```python
from build123d import *

# Parameters (mm, degrees)
BOSS_EXTRUDE1_DEPTH = 2
SKETCH3_R           = 10
CUT_EXTRUDE2_DEPTH  = 2
SKETCH2_R           = 1.75
CUT_EXTRUDE1_DEPTH  = 2
SKETCH4_R           = 1.75
CUT_EXTRUDE3_DEPTH  = 2
CIRPATTERN1_COUNT   = 4


with BuildPart() as part:
    # Sketch1 → Boss-Extrude1 (new body)
    with BuildSketch(Plane(origin=(0, 0, 0), x_dir=(1, 0, 0), z_dir=(0, 1, 0))):
        Polygon((-25, 50), (25, 50), (50, 25), (50, -25), (25, -50), (-25, -50), (-50, -25), (-50, 25), align=None)
    extrude(amount=BOSS_EXTRUDE1_DEPTH)

    # Sketch3 → Cut-Extrude2 (cut)
    with BuildSketch(Plane(origin=(0, 2, 0), x_dir=(1, 0, 0), z_dir=(0, 1, 0))):
        Circle(SKETCH3_R)
    extrude(amount=-CUT_EXTRUDE2_DEPTH, mode=Mode.SUBTRACT)

    # Sketch2 → Cut-Extrude1 (cut)
    with BuildSketch(Plane(origin=(0, 2, 0), x_dir=(1, 0, 0), z_dir=(0, 1, 0))):
        with Locations((-45, 20)):
            Circle(SKETCH2_R)
        with Locations((-45, 12)):
            Circle(SKETCH2_R)
        with Locations((-45, 4)):
            Circle(SKETCH2_R)
        with Locations((-45, -4)):
            Circle(SKETCH2_R)
        with Locations((-45, -12)):
            Circle(SKETCH2_R)
        with Locations((-45, -20)):
            Circle(SKETCH2_R)
    cut_extrude1 = extrude(amount=-CUT_EXTRUDE1_DEPTH, mode=Mode.SUBTRACT)

    # Sketch4 → Cut-Extrude3 (cut)
    with BuildSketch(Plane(origin=(0, 2, 0), x_dir=(1, 0, 0), z_dir=(0, 1, 0))):
        with Locations((-29.721825407, 38.207106781)):
            Circle(SKETCH4_R)
        with Locations((-24.064971157, 32.550252532)):
            Circle(SKETCH4_R)
        with Locations((-18.408116908, 26.893398282)):
            Circle(SKETCH4_R)
        with Locations((-12.751262658, 21.236544033)):
            Circle(SKETCH4_R)
        with Locations((-7.094408409, 15.579689783)):
            Circle(SKETCH4_R)
        with Locations((-15.579689783, 7.094408409)):
            Circle(SKETCH4_R)
        with Locations((-21.236544033, 12.751262658)):
            Circle(SKETCH4_R)
        with Locations((-26.893398282, 18.408116908)):
            Circle(SKETCH4_R)
        with Locations((-32.550252532, 24.064971157)):
            Circle(SKETCH4_R)
        with Locations((-38.207106781, 29.721825407)):
            Circle(SKETCH4_R)
        Polygon((-30.959262274, 29.898602102), (-16.81712665, 15.756466479), (-15.756466479, 16.81712665), (-29.898602102, 30.959262274), align=None)
        Polygon((-35, 16), (-20, 1), (-20, -1), (-35, -16), align=None)
    cut_extrude3 = extrude(amount=-CUT_EXTRUDE3_DEPTH, mode=Mode.SUBTRACT)

    # CirPattern1: Cut-Extrude1, Cut-Extrude3 ×4 about axis
    cirpattern1_axis = Axis((0, 0, 0), (0, 1, 0))
    for i in range(1, CIRPATTERN1_COUNT):
        add(cut_extrude1.rotate(cirpattern1_axis, i * 360 / CIRPATTERN1_COUNT), mode=Mode.SUBTRACT)
        add(cut_extrude3.rotate(cirpattern1_axis, i * 360 / CIRPATTERN1_COUNT), mode=Mode.SUBTRACT)


solid = part.part
```
Could you check a few things on this model? Use its own coordinates, in mm. Give positions to 0.01 mm unless a question says otherwise; leave off trailing zeros. Order: outer loops, then holes, each group sorted by start corner. A loop starts at its lowest first (then second) coordinate and runs counter-clockwise, first axis right, second up.
Q1. Suppose I cut it at A-A, the plane z = 45. Write out the boundary of the cut face in (x, y).
Q2. Suppose I cut it at B-B, the plane x = 45. Write out the boundary of the cut face in (y, z), and give its area (3 significant figures).
Q3. If I drill on line 1 along Z through (x, y) = (0, 1.6); line 2 along X through (y, z) = (1.3, 39); line 3 along X through (y, z) = (1.4, -32.5), over which ranges is the centre line in solid material (lowest first)?
Q4. Suppose I cut it at C-C, the plane x = 4. Write out the boundary of the cut face in (y, z).
Q5. Suppose I cut it at D-D, the plane y = 1.55. Count the separate pieces of the cut face and the enclosed holes in it, and give its area (3 significant figures).
Solution:
1. outline: (-30, 0) - (-21.75, 0) - (-21.75, 2) - (-30, 2) - close; (-18.25, 0) - (-13.75, 0) - (-13.75, 2) - (-18.25, 2) - close; (-10.25, 0) - (-5.75, 0) - (-5.75, 2) - (-10.25, 2) - close; (-2.25, 0) - (2.25, 0) - (2.25, 2) - (-2.25, 2) - close; (5.75, 0) - (10.25, 0) - (10.25, 2) - (5.75, 2) - close; (13.75, 0) - (18.25, 0) - (18.25, 2) - (13.75, 2) - close; (21.75, 0) - (30, 0) - (30, 2) - (21.75, 2) - close
2. outline: (0, -30) - (2, -30) - (2, -21.75) - (0, -21.75) - close; (0, -18.25) - (2, -18.25) - (2, -13.75) - (0, -13.75) - close; (0, -10.25) - (2, -10.25) - (2, -5.75) - (0, -5.75) - close; (0, -2.25) - (2, -2.25) - (2, 2.25) - (0, 2.25) - close; (0, 5.75) - (2, 5.75) - (2, 10.25) - (0, 10.25) - close; (0, 13.75) - (2, 13.75) - (2, 18.25) - (0, 18.25) - close; (0, 21.75) - (2, 21.75) - (2, 30) - (0, 30) - close
2. area: 78.0 mm2
3. line 1: z = -50 to -35, -20 to -10, 10 to 20, 35 to 50
3. line 2: x = -36 to -31.28, -28.16 to 28.16, 31.28 to 36
3. line 3: x = -42.5 to -25.81, -22.32 to -13.5, 13.5 to 22.32, 25.81 to 42.5
4. outline: (0, -50) - (2, -50) - (2, -46.75) - (0, -46.75) - close; (0, -43.25) - (2, -43.25) - (2, -35) - (0, -35) - close; (0, -23) - (2, -23) - (2, -9.17) - (0, -9.17) - close; (0, 9.17) - (2, 9.17) - (2, 23) - (0, 23) - close; (0, 35) - (2, 35) - (2, 43.25) - (0, 43.25) - close; (0, 46.75) - (2, 46.75) - (2, 50) - (0, 50) - close
5. separate pieces: 1
5. enclosed holes: 73
5. area: 6,680 mm2
